```python
from build123d import *

# Parameters (mm, degrees)
SKETCH_W        = 18.9
SKETCH_H        = 34.8
SKETCH_R        = 1.5
PAD_DEPTH       = 1.5
SKETCH001_W     = 18.9
SKETCH001_H     = 14.8
PAD001_DEPTH    = 8
SKETCH002_R     = 1.2954
POCKET_DEPTH    = 9.501
SKETCH003_R     = 2
POCKET001_DEPTH = 8.5
SKETCH004_R     = 1.5
POCKET002_DEPTH = 1.001
SKETCH005_W     = 18.9
SKETCH005_H     = 14.1486
POCKET003_DEPTH = 4.1246


with BuildPart() as part:
    # Sketch (on Face6 of Binder) → Pad (new body)
    with BuildSketch(Plane.XY.offset(8)):
        with Locations((14.45, 2.6)):
            Rectangle(SKETCH_W, SKETCH_H)
        with Locations((9.45, 17.5)):
            Circle(SKETCH_R, mode=Mode.SUBTRACT)
        with Locations((9.45, 2.5)):
            Circle(SKETCH_R, mode=Mode.SUBTRACT)
        with Locations((19.45, 2.5)):
            Circle(SKETCH_R, mode=Mode.SUBTRACT)
        with Locations((19.45, 17.5)):
            Circle(SKETCH_R, mode=Mode.SUBTRACT)
    extrude(amount=PAD_DEPTH)

    # Sketch001 (on Face9 of Pad) → Pad001 (join)
    with BuildSketch(Plane(origin=(0, 0, 8), x_dir=(1, 0, 0), z_dir=(0, 0, -1))):
        with Locations((14.45, 7.4)):
            Rectangle(SKETCH001_W, SKETCH001_H)
    extrude(amount=PAD001_DEPTH)

    # Sketch002 (on Face15 of Pad001) → Pocket (cut, through all)
    with BuildSketch(Plane(origin=(0, 0, 0), x_dir=(1, 0, 0), z_dir=(0, 0, -1))):
        with Locations((17.573511, 2.15)):
            Circle(SKETCH002_R)
        with Locations((20.6046, 3.9)):
            Circle(SKETCH002_R)
        with Locations((17.573511, 5.65)):
            Circle(SKETCH002_R)
        with Locations((17.573511, 9.15)):
            Circle(SKETCH002_R)
        with Locations((20.6046, 10.9)):
            Circle(SKETCH002_R)
        with Locations((20.6046, 7.4)):
            Circle(SKETCH002_R)
        with Locations((17.573511, 12.65)):
            Circle(SKETCH002_R)
    extrude(amount=-POCKET_DEPTH, mode=Mode.SUBTRACT)

    # Sketch003 (on Face5 of Pocket) → Pocket001 (cut)
    with BuildSketch(Plane.XY.offset(9.5)):
        with Locations((13.573511, -4.65)):
            Circle(SKETCH003_R)
    extrude(amount=-POCKET001_DEPTH, mode=Mode.SUBTRACT)

    # Sketch004 (on Face24 of Pocket001) → Pocket002 (cut, through all)
    with BuildSketch(Plane.XY.offset(1)):
        with Locations((9.45, 2.5)):
            Circle(SKETCH004_R)
    extrude(amount=-POCKET002_DEPTH, mode=Mode.SUBTRACT)

    # Sketch005 (on Face5 of Pocket002) → Pocket003 (cut)
    with BuildSketch(Plane.XY.offset(9.5)):
        with Locations((14.45, -7.7257)):
            Rectangle(SKETCH005_W, SKETCH005_H)
    extrude(amount=-POCKET003_DEPTH, mode=Mode.SUBTRACT)


solid = part.part
```
CAD build for the part. Positions are in the model's coordinates, mm. A direction names the side the tool comes from. Coordinates: 2 decimals unless noted, no trailing zeros. Order: outer loops, then holes, each group sorted by start corner. A loop starts at its lowest first (then second) coordinate and runs counter-clockwise, first axis right, second up. Notation, with made-up numbers: (50.25, 79.25) - (57.25, 79.25) arc R12 cw to (57.25, 92.25) - close; hole circle Ø5 at (75.5, 21). An arc over 180 degrees is marked (long way). Use a Markdown table: item, result. Add a question column.
(1) Flat gauge pins, fed straight in: pin 1 (1 mm diameter, centred on x = 17, z = 6.5, fed in from -Y); pin 2 (4.5 mm diameter, centred on x = 13, y = -3.5, fed in from +Z); pin 3 (4 mm diameter, centred on x = 15, z = 4.5, fed in from +Y). Where does each tip first touch, or does it go through?
(2) Saw through at B-B (y = 17.5). Give the cut face in (x, z).
(3) Which spindle directions (+Z, -Z, +X, -X, +Y, -Y) get a long thin tool onto all of the face, cutting with end or side? Do faces 5 (the face through (14, 0, 4)), 6 (the face through (15.42, -5.42, 3.22)), 7 (the face through (19.31, -7.46, 2.65)). Say none if no direction does.
(4) Pull direction Y, two halves, no side cores. Call faces 1 (the face through (14, -0.651, 7)), 2 (the face through (23.9, -2, 5)), 3 (the face through (14, -5, 1)), 4 (the face through (14, 20, 9)): +Y half, -Y half, draft (parallel to the pull), parting line (faces both ways), or undercut.
(5) Saw through at A-A (y = -12.65). Give the cut face in (x, z), then the cut area to 3 significant figures.
(6) Drill centre lines: line 1 along Y through (x, z) = (19.45, 8.9); line 2 along X through (y, z) = (-12.65, 1.1); line 3 along X through (y, z) = (-6, 2). Where is each one in solid material? Low to high. Write a range as [from, to].
(7) Saw through at C-C (z = 3). Count the separate pieces of the cut face and the enclosed holes in it, then the cut area to 3 significant figures.
Solved:
| question | item | result |
|---|---|---|
| 1 | pin 1 | stops at y = -0.65 |
| 1 | pin 2 | stops at z = 5.38 |
| 1 | pin 3 | stops at y = 0 |
| 2 | outline | (5, 8) - (7.95, 8) - (7.95, 9.5) - (5, 9.5) - close; (10.95, 8) - (17.95, 8) - (17.95, 9.5) - (10.95, 9.5) - close; (20.95, 8) - (23.9, 8) - (23.9, 9.5) - (20.95, 9.5) - close |
| 3 | face 5 | -Z, +X, -X, +Y |
| 3 | face 6 | +Z |
| 3 | face 7 | +Z, -Z |
| 4 | face 1 | -Y half |
| 4 | face 2 | draft |
| 4 | face 3 | undercut |
| 4 | face 4 | +Y half |
| 5 | outline | (5, 0) - (16.28, 0) - (16.28, 5.38) - (5, 5.38) - close; (18.87, 0) - (23.9, 0) - (23.9, 5.38) - (18.87, 5.38) - close |
| 5 | area | 87.7 mm² |
| 6 | line 1 | y = [-0.65, 1], [4, 16], [19, 20] |
| 6 | line 2 | x = [5, 16.28], [18.87, 23.9] |
| 6 | line 3 | x = [5, 12.1], [15.05, 16.33], [18.82, 23.9] |
| 7 | separate pieces | 1 |
| 7 | enclosed holes | 8 |
| 7 | area | 230 mm² |
